Design review of the part built by this model. Coordinates are the model's own, in mm. A direction names the side the tool comes from. Give positions to 0.01 mm unless a question says otherwise; leave off trailing zeros. Order: outer loops, then holes, each group sorted by start corner. A loop starts at its lowest first (then second) coordinate and runs counter-clockwise, first axis right, second up. Notation, with made-up numbers: M -23,37.25 L 5,37.25 A5 cw 5,45.25 Z; hole C 27.5,-15.5 d8. An arc over 180 degrees is marked long. Put each result on its own line as item: value. Start each with the question number.
Autodesk Inventor part; units mm, degrees
ref_plane "YZ Plane" through (0, 0, 0) normal (1, 0, 0) x (0, 1, 0)
ref_plane "XZ Plane" through (0, 0, 0) normal (0, 1, 0) x (-1, 0, 0)
ref_plane "XY Plane" through (0, 0, 0) normal (0, 0, 1) x (1, 0, 0)
sketch "Sketch1" plane through (0, 0, 0) normal (1, 0, 0) x (0, 1, 0)
  line L0 (0, 0) -> (42, 0)
  line L1 (42, 0) -> (42, 42)
  line L2 (42, 42) -> (0, 42)
  line L3 (0, 42) -> (0, 0)
  dimension "d0" = 42
  dimension "d1" = 42
extrude "Extrusion1" add sketch "Sketch1" against normal blind 47
sketch "Sketch2" plane through (0, 0, 0) normal (1, 0, 0) x (0, 0, -1)
  line L0 (-42, 42) -> (0, 42) construction
  line L1 (-21, 42) -> (-21, 0) construction
  line L2 (0, 0) -> (-42, 0) construction
  circle A0 centre (-21, 21) radius 11
  circle A1 centre (-21, 21) radius 4
  dimension "d4" = 22
  dimension "d5" = 8
extrude "Extrusion2" add sketch "Sketch2" along normal blind 2
sketch "Sketch3" plane through (0, 21, 21) normal (1, 0, 0) x (0, 0, -1)
  circle A0 centre (0, 0) radius 4
  circle A1 centre (0, 0) radius 2.5
  point P0 (21, -21)
  dimension "d8" = 5
extrude "Extrusion3" add sketch "Sketch3" along normal blind 22 contours A1
chamfer "Chamfer1" distance 5 angle 45 4 edges at (-23.5, 42, 42) (-23.5, 42, 0) (-23.5, 0, 42) (-23.5, 0, 0)
sketch "Sketch4" plane through (0, 0, 0) normal (1, 0, 0) x (0, 0, -1)
  line L0 (-35.375, 35.3745) -> (-6.625, 35.3745) construction
  line L1 (-6.625, 35.3745) -> (-6.625, 6.6245) construction
  line L2 (-6.625, 6.6245) -> (-35.375, 6.6245) construction
  line L3 (-35.375, 6.6245) -> (-35.375, 35.3745) construction
  line L4 (-42, 37) -> (-42, 5) construction
  line L5 (-5, 42) -> (-37, 42) construction
  circle A0 centre (-6.625, 35.3745) radius 1.25
  circle A1 centre (-35.375, 35.3745) radius 1.25
  circle A2 centre (-35.375, 6.6245) radius 1.25
  circle A3 centre (-6.625, 6.6245) radius 1.25
  point P0 (0, 0)
  dimension "d14" = 28.75
  dimension "d15" = 28.75
  dimension "d16" = 6.625
  dimension "d17" = 6.6255
  dimension "d18" = 2.5
  dimension "d19" = 2.5
  dimension "d20" = 2.5
  dimension "d21" = 2.5
extrude "Extrusion4" cut sketch "Sketch4" against normal blind 5
sketch "Sketch5" plane through (0, 0, 0) normal (1, 0, 0) x (0, 0, -1)
  line L0 (-46, 42) -> (4, 42)
  line L1 (4, 42) -> (4, -9)
  line L2 (4, -9) -> (-46, -9)
  line L3 (-46, -9) -> (-46, 42)
  line L4 (-5, 42) -> (-37, 42) construction
  line L5 (-42, 37) -> (-42, 5) construction
  circle A0 centre (-21, 21) radius 11
  circle A1 centre (-35.375, 35.3745) radius 1.25
  circle A2 centre (-6.625, 35.3745) radius 1.25
  circle A3 centre (-6.625, 6.6245) radius 1.25
  circle A4 centre (-35.375, 6.6245) radius 1.25
  circle A5 centre (-35.375, 35.3745) radius 2.3338
  circle A6 centre (-6.625, 35.3745) radius 1.7372
  circle A7 centre (-35.375, 6.6245) radius 2.4239
  circle A8 centre (-6.625, 6.6245) radius 2.2788
  circle A9 centre (-21, 21) radius 12
  point P0 (0, 0)
  dimension "d24" = 50
  dimension "d25" = 51
  dimension "d26" = 4
  dimension "d27" = 0
  dimension "d28" = 1.0838
  dimension "d29" = 0.4872
  dimension "d30" = 1.1739
  dimension "d31" = 1.0288
  dimension "d32" = 1
extrude "Extrusion5" add sketch "Sketch5" along normal blind 2.75 contours L0 L1 L2 L3
sketch "Sketch6" plane through (0, 0, 0) normal (-1, 0, 0) x (0, 0, 1)
  line L0 (42, 37) -> (37, 42)
  line L1 (42, 37) -> (42, 5)
  line L2 (37, 0) -> (42, 5)
  line L3 (37, 0) -> (5, 0)
  line L4 (0, 5) -> (5, 0)
  line L5 (0, 5) -> (0, 37)
  line L6 (5, 42) -> (0, 37)
  line L7 (-4, 42) -> (5, 42)
  line L8 (-4, -9) -> (-4, 42)
  line L9 (46, -9) -> (-4, -9)
  line L10 (46, 42) -> (46, -9)
  line L11 (37, 42) -> (46, 42)
  line L12 (-4, -6.25) -> (46, -6.25)
  line L13 (46, 42) -> (46, -9)
  point P0 (0, 0)
  dimension "d35" = 2.75
extrude "Extrusion6" add sketch "Sketch6" along normal blind 51 contours L10 L9 L8 L12
sketch "Sketch7" plane through (2.75, -9, -4) normal (0, -1, 0) x (1, 0, 0)
  line L0 (-42.625, 9.625) -> (-13.625, 9.625) construction
  line L1 (-42.625, 7.5) -> (-13.625, 7.5)
  line L2 (-13.625, 11.75) -> (-42.625, 11.75)
  arc A0 (-42.625, 11.75) -> (-42.625, 7.5) centre (-42.625, 9.625) ccw
  arc A1 (-13.625, 7.5) -> (-13.625, 11.75) centre (-13.625, 9.625) ccw
  line L3 (-53.75, 0) -> (0, 0)
  line L4 (-53.75, 0) -> (-53.75, 50)
  line L5 (-53.75, 25) -> (0, 25) construction
  line L6 (0, 50) -> (0, 0) construction
  line L7 (-42.625, 42.5) -> (-13.625, 42.5)
  line L8 (-13.625, 38.25) -> (-42.625, 38.25)
  arc A2 (-42.625, 42.5) -> (-42.625, 38.25) centre (-42.625, 40.375) ccw
  arc A3 (-13.625, 38.25) -> (-13.625, 42.5) centre (-13.625, 40.375) ccw
  point P0 (-2.75, 4)
  point P1 (-28.125, 9.625)
  dimension "d38" = 29
  dimension "d39" = 4.25
  dimension "d40" = 7.5
  dimension "d41" = 11.125
extrude "Extrusion7" cut sketch "Sketch7" against normal up to next
properties part number "Nema 17 CNC Kit Stepper Motor"
1. Machinability: for faces 5 (the flat face through (-26, -8, 38.5)), 6 (the flat face through (-23, 21, 0)), 7 (the flat face through (-5, 35, 7)), which of the approach directions +Z, -Z, +X, -X, +Y, -Y give a long, thin tool a straight path to every point of the face, cutting with its end or side? Answer none if there is none.
2. Consider section C-C on z = 21. Give the boundary of the cut face in (x, y).
3. Consider section B-B on y = 21. Give the boundary of the cut face in (x, z).
4. Consider section A-A on x = -32.5. Give the boundary of the cut face in (y, z), then the cut area to 3 significant figures.
5. To check wall thickness, follow probe 1 along Z at (x, y) = (2, 35.5); probe 2 along Y at (x, z) = (1, 21); probe 3 along Y at (x, z) = (-21, 30.5). State the ranges of each line that lie inside material, in increasing order.
6. The part is to be moulded in two halves that separate along Y. For faces 1 (the flat face through (-24, 40, 39)), 2 (the cylindrical face through (-42, -7.6, 5.7)), 3 (the flat face through (0, 8, 6)), 4 (the cylindrical face through (0.986, 30.759, 15.924)), say which applies: +Y half, -Y half, draft (parallel to the pull), parting line (faces both ways), or undercut.
7. Consider section D-D on x = 9.5. Give the boundary of the cut face in (y, z), then the cut area to 3 significant figures.
8. Insertion check: pin 1 (4 mm diameter, centred on y = 35.37, z = 6.62, fed in from -X); pin 2 (8 mm diameter, centred on y = 34, z = 29.5, fed in from +X); pin 3 (2 mm diameter, centred on y = 35.37, z = 6.62, fed in from +X). Each pin has a flat end and moves straight along its axis. Give the tip position at first contact, or say it passes through.
Returned:
1. face 5: -Y
1. face 6: -Z, -X, +Y
1. face 7: +X
2. outline: M -51,-9 L 2.75,-9 L 2.75,9 L 0,9 L 0,10 L 2,10 L 2,17 L 0,17 L 0,18.5 L 22,18.5 L 22,23.5 L 0,23.5 L 0,25 L 2,25 L 2,32 L 0,32 L 0,33 L 2.75,33 L 2.75,42 L -47,42 L -47,0 L 0,0 L 0,-6.25 L -51,-6.25 Z
3. outline: M -47,0 L 0,0 L 0,-4 L 2.75,-4 L 2.75,9 L 0,9 L 0,10 L 2,10 L 2,17 L 0,17 L 0,18.5 L 22,18.5 L 22,23.5 L 0,23.5 L 0,25 L 2,25 L 2,32 L 0,32 L 0,33 L 2.75,33 L 2.75,46 L 0,46 L 0,42 L -47,42 Z
4. outline: M -9,-4 L -6.25,-4 L -6.25,3.5 L -9,3.5 Z; M -9,7.75 L -6.25,7.75 L -6.25,34.25 L -9,34.25 Z; M -9,38.5 L -6.25,38.5 L -6.25,46 L -9,46 Z; M 0,5 L 5,0 L 37,0 L 42,5 L 42,37 L 37,42 L 5,42 L 0,37 Z
4. area: 1,830 mm2
5. probe 1: z = -4 to 4.89, 8.36 to 33.04, 37.71 to 46
5. probe 2: y = -9 to 9, 10 to 17, 18.5 to 23.5, 25 to 32, 33 to 42
5. probe 3: y = -9 to -6.25, 0 to 42
6. face 1: +Y half
6. face 2: draft
6. face 3: undercut
6. face 4: undercut
7. outline: C 21,21 d5
7. area: 19.6 mm2
8. pin 1: stops at x = -47
8. pin 2: stops at x = 2.75
8. pin 3: stops at x = -5
